from build123d import *

# Parameters (mm, degrees)
CYLINDER001_W     = 10
CYLINDER001_H     = 10
CYLINDER001_ANGLE = 45
ARRAY_COUNT       = 8
CYLINDER_R        = 12
CYLINDER_DEPTH    = 10


with BuildPart() as array:
    # Cylinder001 → Cylinder001 (revolve)
    with BuildSketch(Plane(origin=(1, 0.25, 0), x_dir=(1, 0, 0), z_dir=(0, -1, 0))):
        with Locations((5, 5)):
            Rectangle(CYLINDER001_W, CYLINDER001_H)
    revolve(axis=Axis((1, 0.25, 0), (0, 0, 1)), revolution_arc=CYLINDER001_ANGLE)

    # Array: Array ×8 about axis
    array_axis = Axis((0, 0, 0), (0, 0, 1))


with BuildPart() as array_1:
    add(array.part)
    for i in range(1, ARRAY_COUNT):
        add(array.part.rotate(array_axis, i * 360 / ARRAY_COUNT))


with BuildPart() as array_2:
    # Array placement: moved
    add(array_1.part.moved(Location((0, 0, 5))))


with BuildPart() as cut:
    # Cylinder → Cylinder (new body)
    with BuildSketch(Plane.XY):
        Circle(CYLINDER_R)
    extrude(amount=CYLINDER_DEPTH)

    # Cut: cut Array
    add(array_2.part, mode=Mode.SUBTRACT)


solid = cut.part
Here's how the part is built. I have some questions about the finished solid (model axes, mm). Round coordinates to 2 decimals unless told otherwise and drop trailing zeros. Order: outer loops, then holes, each group sorted by start corner. A loop starts at its lowest first (then second) coordinate and runs counter-clockwise, first axis right, second up. Notation, with made-up numbers: M 36.25,46.25 L 57.25,46.25 A24 cw 57.25,57.25 Z; hole C -10,35 d4. An arc over 180 degrees is marked long. Return JSON: item names as keys, results as strings. Group by question number.
1. I'm going to push flat-ended pins straight in: pin 1 Ø1 at (x, y) = (-4.5, -6.5) entering from +Z; pin 2 Ø1.5 at (x, z) = (5.5, 1) entering from -Y; pin 3 Ø4 at (y, z) = (4.5, 2.5) entering from +X. Where does each tip first touch, or does it pass through?
2. If we mould it in two halves opening along Y, with no side actions, what happens to faces 1 (the face through (-6, 0.53, 8)), 2 (the face through (-11.99, 0.53, 4.93)), 3 (the face through (0, 0, 0))? For each: pulls with the +Y half, pulls with the -Y half, needs draft (parallel to the pull), parting line crosses it, or undercut.
3. If we section it at A-A on x = -7: List the corners of the cut face in (y, z) for me.
4. If we section it at D-D on y = -8.75: List the corners of the cut face in (x, z) for me.
5. Please list where these lines run through material, in increasing order: probe 1 along X at (y, z) = (5, 6.5); probe 2 along Y at (x, z) = (-3.25, 8); probe 3 along X at (y, z) = (-3.5, 7.5).
6. If we section it at C-C on z = 4.5: List the corners of the cut face in (x, y) for me, then the cut area to 3 significant figures.
7. If we section it at B-B on y = 3: List the corners of the cut face in (x, z) for me, then the cut area to 3 significant figures.
Reply:
{
 "1": {"pin 1": "z = 5", "pin 2": "y = -11.02", "pin 3": "x = 11.74"},
 "2": {"face 1": "undercut", "face 2": "parting line crosses it", "face 3": "needs draft"},
 "3": {"outline": "M -9.75,0 L 9.75,0 L 9.75,10 L 8.38,10 L 8.38,5 L 7.75,5 L 7.75,10 L 6.65,10 L 6.65,5 L 0.53,5 L 0.53,10 L -0.25,10 L -0.25,5 L -6.25,5 L -6.25,10 L -7.35,10 L -7.35,5 L -8.51,5 L -8.51,10 L -9.75,10 Z"},
 "4": {"outline": "M -8.21,0 L 8.21,0 L 8.21,10 L 6.57,10 L 6.57,5 L 0.25,5 L 0.25,10 L -0.53,10 L -0.53,5 L -6.7,5 L -6.7,10 L -8.21,10 Z"},
 "5": {"probe 1": "-10.91 to -9.83, -5.35 to -4.25, -0.25 to 0.53, 4.65 to 5.75, 9.8 to 10.91", "probe 2": "-11.55 to -10.51, -3.6 to -2.5, -0.25 to 0.53, 2.9 to 4, 10.54 to 11.55", "probe 3": "-11.48 to -10.46, -4.25 to -3.15, -0.53 to 0.25, 2.75 to 3.85, 10.43 to 11.48"},
 "6": {"outline": "C 0,0 d24", "area": "452 mm^2"},
 "7": {"outline": "M -11.62,0 L 11.62,0 L 11.62,10 L 10.61,10 L 10.61,5 L 3.75,5 L 3.75,10 L 2.65,10 L 2.65,5 L 0.53,5 L 0.53,10 L -0.25,10 L -0.25,5 L -2.25,5 L -2.25,10 L -3.35,10 L -3.35,5 L -10.57,5 L -10.57,10 L -11.62,10 Z", "area": "141 mm^2"}
}
